The model under review builds one solid part; all positions refer to its coordinate system, in mm. A direction names the side the tool comes from. Coordinates: 2 decimals unless noted, no trailing zeros. Write each loop counter-clockwise with the first axis right and the second up, starting at its lowest first coordinate (ties: lowest second). Pieces come first, ordered by that corner, then holes.
Autodesk Inventor part; units mm, degrees
ref_plane "YZ Plane" through (0, 0, 0) normal (1, 0, 0) x (0, 1, 0)
ref_plane "XZ Plane" through (0, 0, 0) normal (0, 1, 0) x (-1, 0, 0)
ref_plane "XY Plane" through (0, 0, 0) normal (0, 0, 1) x (1, 0, 0)
sketch "Sketch1" plane through (0, 0, 0) normal (0, 0, 1) x (1, 0, 0)
  line L0 (0, 0) -> (87.28, 0)
  line L1 (0, 0) -> (0, 15.7)
  line L2 (87.28, 0) -> (87.28, 15.7)
  line L3 (87.28, 15.7) -> (0, 15.7)
  dimension "d0" = 87.28
  dimension "d1" = 15.7
  dimension "d2" = 15.7
extrude "Extrusion1" add sketch "Sketch1" along normal blind 3
sketch "Sketch2" plane through (0, 0, 0) normal (0, -1, 0) x (1, 0, 0)
  line L0 (87.28, 0) -> (0, 0)
  line L1 (0, 0) -> (0, -297.64)
  line L2 (0, -297.64) -> (87.28, -297.64)
  line L3 (87.28, -297.64) -> (87.28, 0)
  dimension "d5" = 297.64
extrude "Extrusion2" add sketch "Sketch2" against normal blind 3
sketch "Sketch3" plane through (87.28, 0, 3) normal (1, 0, 0) x (0, 0, -1)
  line L0 (0, 15.7) -> (0, 79.2)
  line L1 (0, 79.2) -> (3, 79.2)
  line L2 (3, 15.7) -> (0, 15.7)
  line L3 (3, 79.2) -> (3, 15.7)
  line L4 (3, 3) -> (3, 15.7)
  line L5 (3, 15.7) -> (3, 3)
  line L6 (3, 3) -> (300.64, 3)
  line L7 (300.64, 3) -> (300.64, 79.2)
  line L8 (300.64, 79.2) -> (3, 79.2)
  point P0 (3, 0)
  dimension "d8" = 63.5
extrude "Extrusion3" add sketch "Sketch3" against normal blind 3
fillet "Fillet1" radius 20 1 edges at (85.78, 79.2, 3)
sketch "Sketch4" plane through (0, 0, 3) normal (-1, 0, 0) x (0, 0, 1)
  line L0 (0, 0) -> (0, 59.2)
  line L1 (0, 15.7) -> (0, 79.2)
  line L2 (0, 79.2) -> (-3, 79.2)
  line L3 (0, 15.7) -> (-3, 15.7)
  line L4 (-3, 79.2) -> (-3, 15.7)
  line L5 (-3, 15.7) -> (-3, 3)
  line L6 (-3, 15.7) -> (-3, 3)
  line L7 (-3, 3) -> (-300.64, 3)
  line L8 (-300.64, 0) -> (-300.64, 79.2)
  line L9 (-300.64, 79.2) -> (-300.64, 3)
  line L10 (-300.64, 79.2) -> (-3, 79.2)
  point P0 (-3, 0)
  dimension "d12" = 63.5
  dimension "d13" = 3
extrude "Extrusion4" add sketch "Sketch4" against normal blind 3
fillet "Fillet2" radius 20 1 edges at (1.5, 79.2, 3)
sketch "Sketch5" plane through (87.28, 0, -297.64) normal (0, 0, -1) x (-1, 0, 0)
  line L0 (0, 79.2) -> (3, 79.2)
  line L1 (3, 3) -> (84.28, 3)
  line L2 (3, 79.2) -> (84.28, 79.2)
  line L3 (84.28, 79.2) -> (84.28, 3)
  line L4 (84.28, 3) -> (3, 3)
  line L5 (3, 3) -> (3, 79.2)
  point P0 (87.28, 0)
extrude "Extrusion5" add sketch "Sketch5" against normal blind 3
sketch "Sketch6" plane through (87.28, 0, 3) normal (1, 0, 0) x (0, 0, -1)
  line L0 (300.64, 0) -> (300.64, 79.2)
  line L1 (300.64, 3) -> (288.125, 3)
  line L2 (300.64, 0) -> (0, 0)
  line L3 (300.64, 3) -> (300.64, 15.7)
  line L4 (288.125, 3) -> (288.125, 15.7)
  line L5 (288.125, 15.7) -> (300.64, 15.7)
  point P0 (3, 0)
  dimension "d19" = 3
  dimension "d20" = 12.515
  dimension "d21" = 12.7
extrude "Extrusion6" cut sketch "Sketch6" against normal blind 3
sketch "Sketch7" plane through (87.28, 0, -297.64) normal (0, 0, -1) x (-1, 0, 0)
  line L0 (0, 15.7) -> (3, 15.7)
  line L1 (3, 15.7) -> (12.515, 15.7)
  line L2 (3, 15.7) -> (84.28, 15.7)
  line L3 (12.515, 15.7) -> (12.515, 3)
  line L4 (3, 3) -> (84.28, 3)
  line L5 (0, 3) -> (3, 3)
  line L6 (3, 3) -> (12.515, 3)
  line L7 (3, 15.7) -> (3, 3)
  line L8 (3, 15.7) -> (3, 3)
  point P0 (87.28, 0)
  dimension "d24" = 9.515
extrude "Extrusion7" cut sketch "Sketch7" against normal blind 3
sketch "Sketch8" plane through (87.28, 0, -297.64) normal (0, 0, -1) x (-1, 0, 0)
  line L0 (87.28, 0) -> (87.28, 79.2)
  line L1 (87.28, 3) -> (74.765, 3)
  line L2 (87.28, 0) -> (0, 0)
  line L3 (74.765, 3) -> (74.765, 15.7)
  line L4 (74.765, 15.7) -> (87.28, 15.7)
  line L5 (87.28, 15.7) -> (87.28, 3)
  dimension "d27" = 3
  dimension "d28" = 12.515
  dimension "d29" = 12.7
extrude "Extrusion8" cut sketch "Sketch8" against normal blind 3
sketch "Sketch9" plane through (0, 0, -297.64) normal (-1, 0, 0) x (0, 0, 1)
  line L0 (0, 15.7) -> (3, 15.7)
  line L1 (3, 3) -> (3, 15.7)
  line L2 (3, 15.7) -> (3, 3)
  line L3 (12.515, 15.7) -> (0, 15.7)
  line L4 (3, 15.7) -> (12.515, 15.7)
  line L5 (12.515, 15.7) -> (12.515, 3)
  line L6 (12.515, 15.7) -> (12.515, 3)
  line L7 (12.515, 3) -> (3, 3)
  point P0 (297.64, 0)
extrude "Extrusion9" cut sketch "Sketch9" against normal blind 3
sketch "Sketch10" plane through (0, 3, 0) normal (0, 1, 0) x (1, 0, 0)
  circle A0 centre (10, 7) radius 2.125
  circle A1 centre (77.28, 7) radius 2.125
  circle A2 centre (10, 287.64) radius 2.125
  circle A3 centre (77.28, 287.64) radius 2.125
  line L0 (0, 297.64) -> (12.515, 297.64)
  line L1 (0, 285.125) -> (0, 297.64)
  line L2 (87.28, 297.64) -> (87.28, 285.125)
  line L3 (74.765, 297.64) -> (87.28, 297.64)
  line L4 (0, -3) -> (87.28, -3)
  line L5 (0, 297.64) -> (0, -3)
  line L6 (87.28, 297.64) -> (87.28, -3)
  point P0 (0, 0)
  dimension "d34" = 4.25
  dimension "d35" = 4.25
  dimension "d36" = 4.25
  dimension "d37" = 4.25
  dimension "d38" = 10
  dimension "d39" = 10
  dimension "d40" = 10
  dimension "d41" = 10
  dimension "d42" = 10
  dimension "d43" = 10
  dimension "d44" = 10
  dimension "d45" = 10
extrude "Extrusion10" cut sketch "Sketch10" against normal blind 3
properties part number "Hopper"
Item 1: To check wall thickness, follow line 1 along Z through (x, y) = (77.28, 1.6) (3 decimals); line 2 along X through (y, z) = (1.15, -7) (3 decimals); line 3 along X through (y, z) = (61.5, -163). State the ranges of each line that lie inside material, in increasing order.
Solved:
line 1: z = -297.64 to -289.765, -285.515 to -9.125, -4.875 to 3
line 2: x = 0 to 7.875, 12.125 to 75.155, 79.405 to 87.28
line 3: x = 0 to 3, 84.28 to 87.28
Item 2: Machinability: for faces 4 (the face through (4, 15.7, -296)), 5 (the face through (1.521, 73.497, -3.014)), 6 (the face through (85, 15.7, -294)), 7 (the face through (43, 9, 0)), 8 (the face through (43, 0, -149)), which of the approach directions +Z, -Z, +X, -X, +Y, -Y give a long, thin tool a straight path to every point of the face, cutting with its end or side? Answer none if there is none.
Solved:
face 4: -Z, -X
face 5: +Z, +X, -X, +Y
face 6: -Z, +X
face 7: +Y
face 8: +Z, -Z, +X, -X, -Y
Item 3: Take a section at C-C, the plane y = 26. Write out the cut boundary in (x, z), plus the area to 3 significant figures.
Solved:
outline: (0, -297.64) - (87.28, -297.64) - (87.28, 3) - (84.28, 3) - (84.28, -294.64) - (3, -294.64) - (3, 3) - (0, 3) - close
area: 2,050 mm2
Item 4: For pin 1 (0.9 mm diameter, centred on x = 50.5, z = 2, fed in from +Y); pin 2 (6 mm diameter, centred on y = 66, z = -99, fed in from -X); pin 3 (3 mm diameter, centred on x = 62.5, z = -92.5, fed in from +Y); pin 4 (2.5 mm diameter, centred on y = 11, z = -297, fed in from +X) (3 decimals), all flat-tipped, find the tip position at first contact; note any pin that passes through.
Solved:
pin 1: stops at y = 15.7
pin 2: stops at x = 0
pin 3: stops at y = 3
pin 4: stops at x = 74.765
Item 5: Take a section at B-B, the plane z = -163.5. Write out the cut boundary in (x, y).
Solved:
outline: (0, 0) - (87.28, 0) - (87.28, 79.2) - (84.28, 79.2) - (84.28, 3) - (3, 3) - (3, 79.2) - (0, 79.2) - close
Item 6: Take a section at A-A, the plane y = 13. Write out the cut boundary in (x, z) (3 decimals), plus the area to 3 significant figures.
Solved:
outline: (0, -285.125) - (3, -285.125) - (3, 0) - (84.28, 0) - (84.28, -285.125) - (87.28, -285.125) - (87.28, 3) - (0, 3) - close; (12.515, -297.64) - (74.765, -297.64) - (74.765, -294.64) - (12.515, -294.64) - close
area: 2,160 mm2
Item 7: Mouldability with a two-part tool opening along X and no side actions: class faces 1 (the face through (44, 42, -294.64)), 2 (the face through (0, 39, -149)), 3 (the face through (44, 40, -297.64)) as pulls with the +X half, pulls with the -X half, needs draft (parallel to the pull), parting line crosses it, or undercut.
Solved:
face 1: undercut
face 2: pulls with the -X half
face 3: needs draft
